Work out the finished part from the listing and answer in its coordinate system (mm). A direction names the side the tool comes from. Coordinates: 2 decimals unless noted, no trailing zeros. Write each loop counter-clockwise with the first axis right and the second up, starting at its lowest first coordinate (ties: lowest second). Pieces come first, ordered by that corner, then holes. Notation, with made-up numbers: (-14, 36) - (41, 36) arc R10 cw to (41, 41) - close; hole circle Ø1 at (-31.75, 71.25). An arc over 180 degrees is marked (long way). Use a Markdown table: item, result. Add a question column.
(1) A tool of negligible diameter and unlimited length cuts with its end or side. For faces 1 (the face through (64.971, 26.052, 246.5)), 2 (the face through (-76, 70, 449)), 3 (the face through (-227, 1, 350)), 4 (the face through (-219.983, -1.539, 449.3)), from which of +Z, -Z, +X, -X, +Y, -Y can it reach the whole face along a straight path? Write none if from no direction.
(2) Given pin 1 Ø8 at (y, z) = (-19, 74.5) entering from +X; pin 2 Ø6 at (x, y) = (-287, -12.5) entering from +Z; pin 3 Ø12 at (x, y) = (-291.5, -5.5) entering from -Z, each flat-ended and moving along its own axis, determine where each tip first touches the part or whether it passes through.
(3) The part is cut by section D-D, the plane y = -51.5. Give the vertices of the cut face in (x, z).
(4) The part is cut by section A-A, the plane y = 0. Give the vertices of the cut face in (x, z).
(5) The part is cut by section B-B, the plane z = 257. Give the vertices of the cut face in (x, y), then the cut area to 3 significant figures.
(6) For a pull along X with two mould halves and no side action, classify faces 5 (the face through (-369.983, 1.539, 375.35)), 6 (the face through (-74, -70, 449)), 7 (the face through (-75, 6, 400)) as released by +X, released by -X, zero draft, split by the parting line, or undercut.
(7) Find the intervals of material crossed by line 1 (X direction, y = -6.5, z = 378); line 2 (Z direction, x = -193, y = -13); line 3 (Z direction, x = -232.5, y = 59.5), in increasing order. Write a range as from..to.
(8) The part is cut by section C-C, the plane x = -233.5. Give the vertices of the cut face in (y, z).
from build123d import *

# Parameters (mm, degrees)
SZKIC1_R                    = 70
DODANIE_WYCI_GNI_CIE1_DEPTH = 400
DODANIE_WYCI_GNI_CIE2_DEPTH = 100
DODANIE_WYCI_GNI_CIE3_DEPTH = 50


with BuildPart() as part:
    # Szkic1 → Dodanie-wyci_gni_cie1 (new body)
    with BuildSketch(Plane.XY):
        Circle(SZKIC1_R)
    extrude(amount=DODANIE_WYCI_GNI_CIE1_DEPTH)

    # Szkic2 → Dodanie-wyci_gni_cie2 (add)
    with BuildSketch(Plane.XY.offset(400)):
        with BuildLine():
            Line((0, -70), (-150, -70))
            ThreePointArc((-150, -70), (-220, 0), (-150, 70))
            Line((-150, 70), (0, 70))
            ThreePointArc((0, 70), (70, 0), (0, -70))
        make_face()
    extrude(amount=DODANIE_WYCI_GNI_CIE2_DEPTH)

    # Szkic3 → Dodanie-wyci_gni_cie3 (add)
    with BuildSketch(Plane(origin=(0, 0, 400), x_dir=(-1, 0, 0), z_dir=(0, 0, -1))):
        with BuildLine():
            Line((150, 70), (300, 70))
            ThreePointArc((300, 70), (370, 0), (300, -70))
            Line((300, -70), (150, -70))
            ThreePointArc((150, -70), (80, 0), (150, 70))
        make_face()
    extrude(amount=DODANIE_WYCI_GNI_CIE3_DEPTH)


solid = part.part
Model answer:
| question | item | result |
|---|---|---|
| 1 | face 1 | -Z |
| 1 | face 2 | +Z, -Z, +X, -X, +Y |
| 1 | face 3 | -Z, -X, +Y, -Y |
| 1 | face 4 | +Z, -X |
| 2 | pin 1 | x = 68.37 |
| 2 | pin 2 | z = 400 |
| 2 | pin 3 | z = 350 |
| 3 | outline | (-347.41, 350) - (-102.59, 350) - (-102.59, 400) - (-47.41, 400) - (-47.41, 0) - (47.41, 0) - (47.41, 500) - (-197.41, 500) - (-197.41, 400) - (-347.41, 400) - close |
| 4 | outline | (-370, 350) - (-80, 350) - (-80, 400) - (-70, 400) - (-70, 0) - (70, 0) - (70, 500) - (-220, 500) - (-220, 400) - (-370, 400) - close |
| 5 | outline | circle Ø140 at (0, 0) |
| 5 | area | 15,400 mm^2 |
| 6 | face 5 | released by -X |
| 6 | face 6 | zero draft |
| 6 | face 7 | undercut |
| 7 | line 1 | -369.7..-80.3, -69.7..69.7 |
| 7 | line 2 | 350..500 |
| 7 | line 3 | 350..400 |
| 8 | outline | (-70, 350) - (70, 350) - (70, 400) - (-70, 400) - close |
